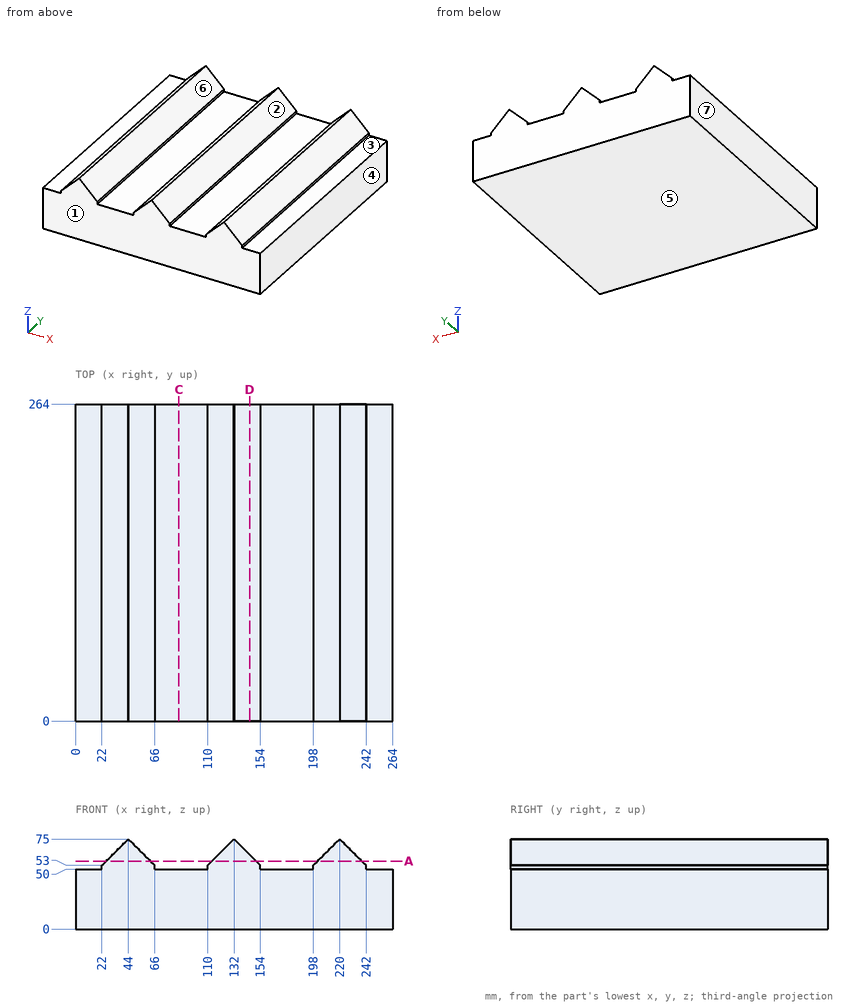
Here's the drawing with two shaded views (mm, measured from the low corner). I have some questions. A direction names the side the tool comes from. Coordinates: 2 decimals unless noted, no trailing zeros. Write each loop counter-clockwise with the first axis right and the second up, starting at its lowest first coordinate (ties: lowest second). Pieces come first, ordered by that corner, then holes. Notation, with made-up numbers: (0, 31) -> (17, 31) arc R17 ccw to (17, 63) -> close; hole circle Ø9 at (-29, -19.75). An arc over 180 degrees is marked (long way). One line per question, with ' | ' between items. Start each with the question number.
1. For the marked faces 1, 2 and 3, which set-ups out of +Z, -Z, +X, -X, +Y, -Y let a thin tool reach every point of the face, with its end or its side?
2. If we section it at D-D (x = 145): Please give me the cut outline in (y, z).
3. Will these pins go through, and if not, where does the flat tip stop? P1, Ø1.5, axis at y = 177.5, z = 51, coming from the -X side; P2, Ø12, axis at x = 56.5, y = 203.5, coming from the -Z side; P3, Ø22, axis at x = 176, y = 83.5, coming from the +Z side; P4, Ø0.9, axis at y = 186, z = 51.5, coming from the +X side.
4. If we section it at C-C (x = 86): Please give me the cut outline in (y, z), and give its area (3 significant figures).
5. If we section it at A-A (z = 56.5): Please give me the cut outline in (x, y), and give its area (3 significant figures).
6. Please list where these lines run through material, in increasing order: line 1 along X through (y, z) = (177.5, 59.5); line 2 along Z through (x, y) = (73.5, 237); line 3 along X through (y, z) = (203.5, 64.5).
7. Thinking about a two-plate mould opening in X: for the marked faces 4, 5, 6 and 7, which applies, pulls with the +X half, pulls with the -X half, needs draft (parallel to the pull), parting line crosses it, or undercut?
Return value:
1) face 1: +Z, -Z, +X, -X, -Y | face 2: +Z, +Y, -Y | face 3: +Z, +X, +Y, -Y
2) outline: (0, 0) -> (264, 0) -> (264, 62) -> (0, 62) -> close
3) P1: stops at x = 22 | P2: stops at z = 0 | P3: stops at z = 50 | P4: stops at x = 242
4) outline: (0, 0) -> (264, 0) -> (264, 50) -> (0, 50) -> close | area: 13,200 mm²
5) outline: (25.5, 0) -> (62.5, 0) -> (62.5, 264) -> (25.5, 264) -> close; (113.5, 0) -> (150.5, 0) -> (150.5, 264) -> (113.5, 264) -> close; (201.5, 0) -> (238.5, 0) -> (238.5, 264) -> (201.5, 264) -> close | area: 29,300 mm²
6) line 1: x = 28.5 to 59.5, 116.5 to 147.5, 204.5 to 235.5 | line 2: z = 0 to 50 | line 3: x = 33.5 to 54.5, 121.5 to 142.5, 209.5 to 230.5
7) face 4: pulls with the +X half | face 5: needs draft | face 6: undercut | face 7: pulls with the -X half
